Geometry: final body of the model. Coordinates: model frame, mm. Round coordinates to 2 decimals unless told otherwise and drop trailing zeros. Loops run counter-clockwise (first coordinate to the right, second up) from the corner with the lowest first, then second, coordinate; pieces in that order, holes last. Notation, with made-up numbers: (21, -9.5) - (62, -9.5) arc R38 ccw to (62, 28.5) - close; hole circle Ø10 at (-38.75, 25). An arc over 180 degrees is marked (long way). Answer as a JSON object with one key per item and string values. Group by question number.
Item 1: First-contact query: pin 1 (5 mm diameter, centred on x = 69.83, y = -69.83, fed in from -Z); pin 2 (1.9 mm diameter, centred on x = 7, z = 1.5, fed in from -Y). Flat tips, straight axial feed; report the tip coordinate or a pass-through.
Item 2: Section C-C (z = 2.6). Count the separate pieces of the cut face and the enclosed holes in it, plus the area to 3 significant figures.
Item 3: Line query: line 1 (Y direction, x = 69.83, z = 1.2); line 2 (Y direction, x = 6.72, z = 1.95); line 3 (Y direction, x = 0, z = 0.75). Output: solid intervals per line, ascending.
Item 4: Section D-D (x = -15). Return the cut outline in (y, z) (3 decimals).
Item 5: Section B-B (y = 63.5). Return the cut outline in (x, z) (3 decimals).
Item 6: Section A-A (y = 0). Return the cut outline in (x, z) (3 decimals).
```python
from build123d import *

# Parameters (mm, degrees)
SKETCH3_W               = 152.4
SKETCH3_H               = 152.4
BOSS_EXTRUDE3_DEPTH     = 3.175
MOTOR_CUT_OUT_DEPTH     = 4.175
SKETCH20_R              = 2.9718
BOLT_HOLES_DEPTH        = 1
BOLT_HOLES_DEPTH_BACK   = 4.175
EDGE_CUT_OUT_DEPTH      = 3.175
FILLET2_R               = 6.35
MIRROR5_COPY_1_DEPTH    = 3.175
FILLET3_R               = 6.35
FILLET4_R               = 6.35
FILLET12_R              = 3
SKETCH27_R              = 1.1
MOTOR_SCREWS_HOLE_DEPTH = 4.175


with BuildPart() as part:
    # Sketch3 → Boss-Extrude3 (new body)
    with BuildSketch(Plane.XY):
        Rectangle(SKETCH3_W, SKETCH3_H)
    extrude(amount=BOSS_EXTRUDE3_DEPTH)

    # Sketch13 → Motor Cut Out (cut, through all)
    with BuildSketch(Plane(origin=(0.106889783, -2.03090588, 3.175), x_dir=(1, 0, 0), z_dir=(0, 0, 1))):
        with BuildLine():
            Line((5.483280161, 7.105597989), (10.893110217, 7.105597989))
            Line((10.893110217, 7.105597989), (10.893110217, -2.894402011))
            Line((10.893110217, -2.894402011), (5.483280161, -3.043786229))
            ThreePointArc((5.483280161, -3.043786229), (-7.656889783, 2.03090588), (5.483280161, 7.105597989))
        make_face()
    extrude(amount=-MOTOR_CUT_OUT_DEPTH, mode=Mode.SUBTRACT)

    # Sketch20 → Bolt Holes (cut, two sides)
    with BuildSketch(Plane.XY.offset(3.175)) as bolt_holes_sk:
        with Locations((-69.83, 69.83)):
            Circle(SKETCH20_R)
        with Locations((69.83, 69.83)):
            Circle(SKETCH20_R)
        with Locations((69.83, -69.83)):
            Circle(SKETCH20_R)
        with Locations((-69.83, -69.83)):
            Circle(SKETCH20_R)
    extrude(amount=BOLT_HOLES_DEPTH, mode=Mode.SUBTRACT)
    extrude(bolt_holes_sk.sketch, amount=-BOLT_HOLES_DEPTH_BACK, mode=Mode.SUBTRACT)

    # Sketch25 → Edge cut out (cut)
    with BuildSketch(Plane.XY.offset(3.175)):
        with BuildLine():
            Line((-76.2, 50.8), (-76.2, -50.8))
            ThreePointArc((-76.2, -50.8), (-46.628854397, 0), (-76.2, 50.8))
        make_face()
    edge_cut_out = extrude(amount=-EDGE_CUT_OUT_DEPTH, mode=Mode.SUBTRACT)

    # Fillet2
    fillet2_edges = [part.edges().sort_by_distance(p)[0] for p in [
        (-76.2, -50.8, 1.5875),
        (-76.2, 50.8, 1.5875),
        (-76.2, -76.2, 1.5875),
        (-76.2, 76.2, 1.5875),
    ]]
    fillet(fillet2_edges, radius=FILLET2_R)

    # Mirror4: Edge cut out across plane
    add(edge_cut_out.mirror(Plane(origin=(0, 0, 0), x_dir=(0, 0, 1), z_dir=(0.707106781, -0.707106781, 0))), mode=Mode.SUBTRACT)

    # Mirror5: Edge cut out across plane
    add(edge_cut_out.mirror(Plane(origin=(0, 0, 0), x_dir=(0, 0, 1), z_dir=(-0.707106781, -0.707106781, 0))), mode=Mode.SUBTRACT)

    # Mirror5 copy 1 sketch → Mirror5 copy 1 (cut)
    with BuildSketch(Plane(origin=(0, 0, 3.175), x_dir=(-1, 0, 0), z_dir=(0, 0, 1))):
        with BuildLine():
            Line((-76.2, 50.8), (-76.2, -50.8))
            ThreePointArc((-76.2, -50.8), (-46.628854397, 0), (-76.2, 50.8))
        make_face()
    extrude(amount=-MIRROR5_COPY_1_DEPTH, mode=Mode.SUBTRACT)

    # Fillet3
    fillet3_edges = [part.edges().sort_by_distance(p)[0] for p in [
        (76.2, -76.2, 1.5875),
        (76.2, 76.2, 1.5875),
        (-50.8, -76.2, 1.5875),
        (50.8, -76.2, 1.5875),
        (76.2, 50.8, 1.5875),
        (76.2, -50.8, 1.5875),
    ]]
    fillet(fillet3_edges, radius=FILLET3_R)

    # Fillet4
    fillet4_edges = [part.edges().sort_by_distance(p)[0] for p in [
        (50.8, 76.2, 1.5875),
        (-50.8, 76.2, 1.5875),
    ]]
    fillet(fillet4_edges, radius=FILLET4_R)

    # Fillet12
    fillet12_edges = [part.edges().sort_by_distance(p)[0] for p in [
        (11, 5.074692109, 1.5875),
        (11, -4.925307891, 1.5875),
    ]]
    fillet(fillet12_edges, radius=FILLET12_R)

    # Sketch27 → Motor screws hole (cut, through all)
    with BuildSketch(Plane.XY.offset(3.175)):
        with Locations((6.72, -6.72)):
            Circle(SKETCH27_R)
        with Locations((6.72, 6.72)):
            Circle(SKETCH27_R)
        with Locations((-6.72, 6.72)):
            Circle(SKETCH27_R)
        with Locations((-6.72, -6.72)):
            Circle(SKETCH27_R)
    extrude(amount=-MOTOR_SCREWS_HOLE_DEPTH, mode=Mode.SUBTRACT)


solid = part.part
```
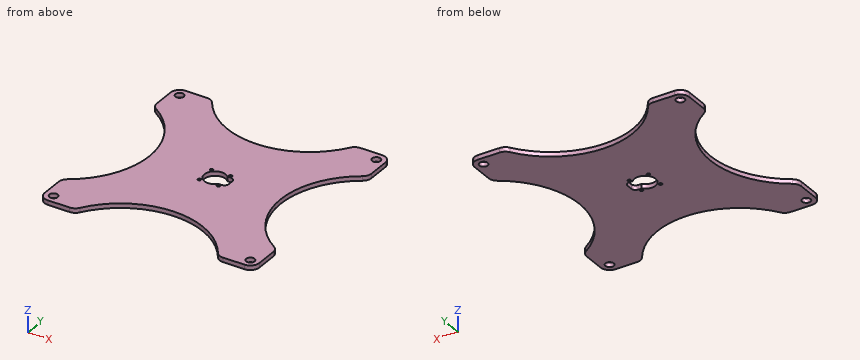
Values:
{
 "1": {"pin 1": "passes through", "pin 2": "stops at y = -47.17"},
 "2": {"separate pieces": "1", "enclosed holes": "9", "area": "14,300 mm^2"},
 "3": {"line 1": "y = -76.2 to -72.8, -66.86 to -46.61, 46.61 to 66.86, 72.8 to 76.2", "line 2": "y = -47.02 to -7.82, -5.62 to -5.04, 5.07 to 5.62, 7.82 to 47.02", "line 3": "y = -46.63 to -7.55, 7.55 to 46.63"},
 "4": {"outline": "(-48.587, 0) - (48.587, 0) - (48.587, 3.175) - (-48.587, 3.175) - close"},
 "5": {"outline": "(-76.2, 0) - (-41.068, 0) - (-41.068, 3.175) - (-76.2, 3.175) - close; (41.068, 0) - (76.2, 0) - (76.2, 3.175) - (41.068, 3.175) - close"},
 "6": {"outline": "(-46.629, 0) - (-7.55, 0) - (-7.55, 3.175) - (-46.629, 3.175) - close; (11, 0) - (46.629, 0) - (46.629, 3.175) - (11, 3.175) - close"}
}
